Autodesk Inventor part; units mm, degrees
ref_plane "YZ Plane" through (0, 0, 0) normal (1, 0, 0) x (0, 1, 0)
ref_plane "XZ Plane" through (0, 0, 0) normal (0, 1, 0) x (-1, 0, 0)
ref_plane "XY Plane" through (0, 0, 0) normal (0, 0, 1) x (1, 0, 0)
sketch "Sketch1" plane through (0, 0, 0) normal (0, 1, 0) x (-1, 0, 0)
  line L0 (-6.5, 15) -> (6.5, 15)
  line L1 (6.5, 15) -> (6.5, -15)
  line L2 (6.5, -15) -> (-6.5, -15)
  line L3 (-6.5, -15) -> (-6.5, 15)
  line L4 (-6.5, 15) -> (6.5, -15) construction
  line L5 (6.5, 15) -> (-6.5, -15) construction
  line L6 (-1.5, 10) -> (1.5, 10)
  line L7 (1.5, 10) -> (1.5, -10)
  line L8 (1.5, -10) -> (-1.5, -10)
  line L9 (-1.5, -10) -> (-1.5, 10)
  line L10 (-1.5, 10) -> (1.5, -10) construction
  line L11 (1.5, 10) -> (-1.5, -10) construction
  circle A0 centre (0, 0) radius 2.5
  point P0 (-1.5, -2)
  point P1 (-1.5, 2)
  point P2 (1.5, 2)
  point P3 (1.5, -2)
  dimension "d0" = 5
  dimension "d1" = 20
  dimension "d2" = 5
  dimension "d3" = 4
  dimension "d4" = 3
extrude "Extrusion1" add sketch "Sketch1" along normal blind 3
properties part number "Acoplador" material "Brass"
For this review, take the finished solid that the model builds, in its own axes (mm). A direction names the side the tool comes from. Round coordinates to 2 decimals unless told otherwise and drop trailing zeros. Write each loop counter-clockwise with the first axis right and the second up, starting at its lowest first coordinate (ties: lowest second). Pieces come first, ordered by that corner, then holes. Notation, with made-up numbers: (57.25, -37) - (89.25, -37) arc R38 ccw to (89.25, 1) - close; hole circle Ø1 at (58, 9.25). An arc over 180 degrees is marked (long way). Use a Markdown table: item, result.
Q1. Wall thickness on line 1 along X through (y, z) = (0.3, -6.5); line 2 along Z through (x, y) = (2, 0.65); line 3 along Z through (x, y) = (-0.5, 1.5): over which ranges is each line inside the solid? List them lowest first.
Derived:
| item | result |
|---|---|
| line 1 | x = -6.5 to -1.5, 1.5 to 6.5 |
| line 2 | z = -15 to -1.5, 1.5 to 15 |
| line 3 | z = -15 to -10, 10 to 15 |
Q2. We need section A-A (x = 0). Give the boundary of the cut face in (y, z), plus the area to 3 significant figures.
Derived:
| item | result |
|---|---|
| outline | (0, -15) - (3, -15) - (3, -10) - (0, -10) - close; (0, 10) - (3, 10) - (3, 15) - (0, 15) - close |
| area | 30.0 mm2 |
Q3. The part is to be moulded in two halves that separate along Z. For faces 1 (the flat face through (0, 1, -15)), 2 (the flat face through (0, 1, 15)), 3 (the flat face through (-6.5, 1, 0)), 4 (the flat face through (-1.5, 1, 6)), say which applies: pulls with the +Z half, pulls with the -Z half, needs draft (parallel to the pull), parting line crosses it, or undercut.
Derived:
| item | result |
|---|---|
| face 1 | pulls with the -Z half |
| face 2 | pulls with the +Z half |
| face 3 | needs draft |
| face 4 | undercut |
Q4. We need section C-C (z = 7.25). Give the boundary of the cut face in (x, y), plus the area to 3 significant figures.
Derived:
| item | result |
|---|---|
| outline | (-6.5, 0) - (-1.5, 0) - (-1.5, 3) - (-6.5, 3) - close; (1.5, 0) - (6.5, 0) - (6.5, 3) - (1.5, 3) - close |
| area | 30.0 mm2 |
Q5. Machinability: for faces 5 (the flat face through (3, 3, 0)), 6 (the flat face through (-1.5, 1, -6)), which of the approach directions +Z, -Z, +X, -X, +Y, -Y give a long, thin tool a straight path to every point of the face, cutting with its end or side? Answer none if there is none.
Derived:
| item | result |
|---|---|
| face 5 | +Z, -Z, +X, -X, +Y |
| face 6 | +Y, -Y |
Q6. We need section B-B (y = 0.8). Give the boundary of the cut face in (x, z), plus the area to 3 significant figures.
Derived:
| item | result |
|---|---|
| outline | (-6.5, -15) - (6.5, -15) - (6.5, 15) - (-6.5, 15) - close; hole (-1.5, -10) - (1.5, -10) - (1.5, -2) arc R2.5 ccw to (1.5, 2) - (1.5, 10) - (-1.5, 10) - (-1.5, 2) arc R2.5 ccw to (-1.5, -2) - close |
| area | 324 mm2 |
